Part model, mm, in its own coordinate system. A direction names the side the tool comes from. Give positions to 0.01 mm unless a question says otherwise; leave off trailing zeros. Order: outer loops, then holes, each group sorted by start corner. A loop starts at its lowest first (then second) coordinate and runs counter-clockwise, first axis right, second up. Notation, with made-up numbers: (67.25, -9.75) - (114.25, -9.75) arc R12 cw to (114.25, 13.25) - close; hole circle Ø8 at (-18, 30). An arc over 180 degrees is marked (long way). One line per item, written item: value.
Solid Edge part; units mm, degrees
sketch "Sketch1" plane through (0, 0, 0) normal (0, 0, 1) x (1, 0, 0)
  line L0 (32.5, 60) -> (-32.5, 60)
  line L1 (-32.5, 60) -> (-32.5, -60)
  line L2 (-32.5, -60) -> (32.5, -60)
  line L3 (32.5, -60) -> (32.5, 60)
extrude "Protrusion1" add sketch "Sketch1" against normal blind 15
sketch "Sketch2" plane through (0, 0, 0) normal (0, 0, 1) x (0, -1, 0)
  circle A0 centre (-47.5, 21) radius 3.25
  circle A1 centre (-47.5, -21) radius 3.25
  circle A2 centre (47.5, 21) radius 3.25
  circle A3 centre (47.5, -21) radius 3.25
extrude "ExtrudedCutout_1" cut sketch "Sketch2" against normal blind 309.8
sketch "Sketch3" plane through (0, 0, 0) normal (0, 0, 1) x (1, 0, 0)
  line L0 (8.2795, -37.5) -> (5.9795, -33.5163)
  line L1 (5.9795, -33.5163) -> (1.3795, -33.5163)
  line L2 (1.3795, -33.5163) -> (-0.9205, -37.5)
  line L3 (-0.9205, -37.5) -> (1.3795, -41.4837)
  line L4 (1.3795, -41.4837) -> (5.9795, -41.4837)
  line L5 (5.9795, -41.4837) -> (8.2795, -37.5)
  line L6 (18.7, -23.5163) -> (16.4, -27.5)
  line L7 (16.4, -27.5) -> (18.7, -31.4837)
  line L8 (18.7, -31.4837) -> (23.3, -31.4837)
  line L9 (23.3, -31.4837) -> (25.6, -27.5)
  line L10 (25.6, -27.5) -> (23.3, -23.5163)
  line L11 (23.3, -23.5163) -> (18.7, -23.5163)
  line L12 (5.9795, -21.4837) -> (8.2795, -17.5)
  line L13 (8.2795, -17.5) -> (5.9795, -13.5163)
  line L14 (5.9795, -13.5163) -> (1.3795, -13.5163)
  line L15 (1.3795, -13.5163) -> (-0.9205, -17.5)
  line L16 (-0.9205, -17.5) -> (1.3795, -21.4837)
  line L17 (1.3795, -21.4837) -> (5.9795, -21.4837)
extrude "ExtrudedCutout_2" cut sketch "Sketch3" against normal blind 4
sketch "Sketch4" plane through (0, 0, 0) normal (0, 0, 1) x (1, 0, 0)
  circle A0 centre (3.6795, -17.5) radius 2.75
  circle A1 centre (21, -27.5) radius 2.75
  circle A2 centre (3.6795, -37.5) radius 2.75
extrude "ExtrudedCutout_3" cut sketch "Sketch4" against normal blind 54.7
1) Slice it at A-A on x = 21. Write the cut outline in (y, z), then the cut area to 3 significant figures.
Answer:
outline: (-60, -15) - (-50.75, -15) - (-50.75, 0) - (-60, 0) - close; (-44.25, -15) - (-30.25, -15) - (-30.25, -4) - (-31.48, -4) - (-31.48, 0) - (-44.25, 0) - close; (-24.75, -15) - (44.25, -15) - (44.25, 0) - (-23.52, 0) - (-23.52, -4) - (-24.75, -4) - close; (50.75, -15) - (60, -15) - (60, 0) - (50.75, 0) - close
area: 1,510 mm2
2) Slice it at C-C on z = -13. Write the cut outline in (x, y), then the cut area to 3 significant figures.
Answer:
outline: (-32.5, -60) - (32.5, -60) - (32.5, 60) - (-32.5, 60) - close; hole circle Ø6.5 at (-21, -47.5); hole circle Ø6.5 at (-21, 47.5); hole circle Ø5.5 at (3.68, -37.5); hole circle Ø5.5 at (3.68, -17.5); hole circle Ø6.5 at (21, -47.5); hole circle Ø6.5 at (21, 47.5); hole circle Ø5.5 at (21, -27.5)
area: 7,600 mm2
3) Slice it at D-D on z = -2. Write the cut outline in (x, y), then the cut area to 3 significant figures.
Answer:
outline: (-32.5, -60) - (32.5, -60) - (32.5, 60) - (-32.5, 60) - close; hole circle Ø6.5 at (-21, -47.5); hole circle Ø6.5 at (-21, 47.5); hole (-0.92, -37.5) - (1.38, -41.48) - (5.98, -41.48) - (8.28, -37.5) - (5.98, -33.52) - (1.38, -33.52) - close; hole (-0.92, -17.5) - (1.38, -21.48) - (5.98, -21.48) - (8.28, -17.5) - (5.98, -13.52) - (1.38, -13.52) - close; hole (16.4, -27.5) - (18.7, -31.48) - (23.3, -31.48) - (25.6, -27.5) - (23.3, -23.52) - (18.7, -23.52) - close; hole circle Ø6.5 at (21, -47.5); hole circle Ø6.5 at (21, 47.5)
area: 7,500 mm2
4) Wall check: line 1 along Y through (x, z) = (3, -3.75); line 2 along X through (y, z) = (47.5, -4.25); line 3 along X through (y, z) = (-16, -5.5). Give the ranges that are in metal, low to high. Write a range as [from, to].
Answer:
line 1: y = [-60, -41.48], [-33.52, -21.48], [-13.52, 60]
line 2: x = [-32.5, -24.25], [-17.75, 17.75], [24.25, 32.5]
line 3: x = [-32.5, 1.37], [5.98, 32.5]
5) Which spindle directions (+Z, -Z, +X, -X, +Y, -Y) get a long thin tool onto all of the face, cutting with end or side? Do faces 1 (the face through (19.755, -50.502, -7.395)), 2 (the face through (21, -31.484, -2)). Say none if no direction does.
Answer:
face 1: +Z, -Z
face 2: +Z
6) Slice it at B-B on y = 47.5. Write the cut outline in (x, z).
Answer:
outline: (-32.5, -15) - (-24.25, -15) - (-24.25, 0) - (-32.5, 0) - close; (-17.75, -15) - (17.75, -15) - (17.75, 0) - (-17.75, 0) - close; (24.25, -15) - (32.5, -15) - (32.5, 0) - (24.25, 0) - close
7) Two-plate mould, pull along Y, no slides. Class faces 3 (the face through (0, -60, -7)), 4 (the face through (7, -17, -4)), 5 (the face through (0, 1, -15)): pulls with the +Y half, pulls with the -Y half, needs draft (parallel to the pull), parting line crosses it, or undercut.
Answer:
face 3: pulls with the -Y half
face 4: undercut
face 5: needs draft
8) Drop flat-ended pins along their axis: P1, Ø3.5, axis at x = 3.68, y = -17.5, coming from the +Z side; P2, Ø4, axis at x = 5, y = -19, coming from the +Z side. Give the stop position or say it passes through.
Answer:
P1: passes through
P2: stops at z = -4
